```python
from build123d import *

# Parameters (mm, degrees)
BOSS_EXTRUDE1_DEPTH = 3.4
SKETCH3_R           = 1.8
BOSS_EXTRUDE2_DEPTH = 1.6


with BuildPart() as part:
    # Sketch2 → Boss-Extrude1 (new body)
    with BuildSketch(Plane(origin=(0, 0, 0), x_dir=(1, 0, 0), z_dir=(0, 1, 0))):
        with BuildLine():
            Line((-2.165640783, -3), (2.165640783, -3))
            ThreePointArc((2.165640783, -3), (2.61629509, -2.61629509), (3, -2.165640783))
            Line((3, -2.165640783), (3, 2.165640783))
            ThreePointArc((3, 2.165640783), (2.61629509, 2.61629509), (2.165640783, 3))
            Line((2.165640783, 3), (-2.165640783, 3))
            ThreePointArc((-2.165640783, 3), (-2.61629509, 2.61629509), (-3, 2.165640783))
            Line((-3, 2.165640783), (-3, -2.165640783))
            ThreePointArc((-3, -2.165640783), (-2.61629509, -2.61629509), (-2.165640783, -3))
        make_face()
    extrude(amount=BOSS_EXTRUDE1_DEPTH)

    # Sketch3 → Boss-Extrude2 (add)
    with BuildSketch(Plane(origin=(0, 3.4, 0), x_dir=(1, 0, 0), z_dir=(0, 1, 0))):
        with Locations(Location((0, 0, 0), (0, 0, 270))):  # turned: the seam where the file's is
            Circle(SKETCH3_R)
    extrude(amount=BOSS_EXTRUDE2_DEPTH)


solid = part.part
```
Input: part model. Units: mm. Frame: model coordinates. A direction names the side the tool comes from. Give positions to 0.01 mm unless a question says otherwise; leave off trailing zeros. Order: outer loops, then holes, each group sorted by start corner. A loop starts at its lowest first (then second) coordinate and runs counter-clockwise, first axis right, second up. Notation, with made-up numbers: M 18,26.5 L 34,26.5 A22 ccw 34,51.5 Z; hole C 2.5,-2.75 d9. An arc over 180 degrees is marked long. One line per question, with ' | ' between items. Start each with the question number.
1. Material intervals for probe 1 along Y at (x, z) = (-0.7, -2.7); probe 2 along X at (y, z) = (4.05, -1.6); probe 3 along Z at (x, y) = (0.85, 4.05), sorted ascending. Write a range as [from, to].
2. Section query B-B (y = 1.15). Return the cut outline in (x, z), and give its area (3 significant figures).
3. Section query D-D (y = 4). Return the cut outline in (x, z), and give its area (3 significant figures).
4. Section query C-C (x = 1.9). Return the cut outline in (y, z).
5. Section query A-A (z = 0). Return the cut outline in (x, y).
6. Access query for faces 1 (the face through (-1.4, 3.4, -1.4)), 2 (the face through (2.61, 1.68, 2.62)). Directions: +Z, -Z, +X, -X, +Y, -Y. A direction counts if a zero-diameter tool reaches every point of the face in a straight line with its end or side. Return the directions, or none.
7. First-contact query: pin 1 Ø3 at (y, z) = (3.5, -1) entering from -X. Flat tip, straight axial feed; report the tip coordinate or a pass-through.
Here are the results:
1) probe 1: [0, 3.4] | probe 2: [-0.82, 0.82] | probe 3: [-1.59, 1.59]
2) outline: M -3,-2.17 A3.7 ccw -2.17,-3 L 2.17,-3 A3.7 ccw 3,-2.17 L 3,2.17 A3.7 ccw 2.17,3 L -2.17,3 A3.7 ccw -3,2.17 Z | area: 34.8 mm²
3) outline: C 0,0 d3.6 | area: 10.2 mm²
4) outline: M 0,-3 L 3.4,-3 L 3.4,3 L 0,3 Z
5) outline: M -3,0 L 3,0 L 3,3.4 L 1.8,3.4 L 1.8,5 L -1.8,5 L -1.8,3.4 L -3,3.4 Z
6) face 1: +Y | face 2: +Z, +X, +Y, -Y
7) pin 1: x = -3
